```python
from build123d import *

# Parameters (mm, degrees)
CROQUIS1_R              = 17.985951022
SALIENTE_EXTRUIR1_DEPTH = 3


with BuildPart() as part:
    # Croquis1 → Saliente-Extruir1 (new body)
    with BuildSketch(Plane.XY):
        with BuildLine():
            Line((69.938444675, 17.671179984), (59.198401062, 17.671179984))
            Line((59.198401062, 17.671179984), (59.198401062, 32.584255723))
            ThreePointArc((59.198401062, 32.584255723), (65.364018559, 84.900042365), (69.938444675, 32.421179984))
            Line((69.938444675, 32.421179984), (69.938444675, 26.421179984))
            Line((69.938444675, 26.421179984), (64.938444675, 26.421179984))
            Line((64.938444675, 26.421179984), (64.938444675, 23.671179984))
            Line((64.938444675, 23.671179984), (69.938444675, 23.671179984))
            Line((69.938444675, 23.671179984), (69.938444675, 17.671179984))
        make_face()
        with Locations((64.962042446, 58.426202565)):
            Circle(CROQUIS1_R, mode=Mode.SUBTRACT)
    extrude(amount=SALIENTE_EXTRUIR1_DEPTH)


solid = part.part
```
The model under review builds one solid part; all positions refer to its coordinate system, in mm. A direction names the side the tool comes from. Round coordinates to 2 decimals unless told otherwise and drop trailing zeros. Order: outer loops, then holes, each group sorted by start corner. A loop starts at its lowest first (then second) coordinate and runs counter-clockwise, first axis right, second up. Notation, with made-up numbers: (-9, 59) -> (46, 59) arc R12 ccw to (46, 70) -> close; hole circle Ø5 at (37.5, -2.5). An arc over 180 degrees is marked (long way). One line per item, written item: value. Start each with the question number.
Q1. Take a section at A-A (x = 54.5). Write out the cut boundary in (y, z).
Q2. Wall thickness on line 1 (Y direction, x = 57.5, z = 1); line 2 (Y direction, x = 50, z = 0.6); line 3 (X direction, y = 59, z = 1.5): over which ranges is each line inside the solid? List them lowest first.
Q3. Mouldability with a two-part tool opening along Y and no side actions: class faces 1 (the face through (64.938, 25, 1)), 2 (the face through (59.198, 25, 1)), 3 (the face through (65, 17.671, 1)) as released by +Y, released by -Y, zero draft, split by the parting line, or undercut.
Q4. Take a section at B-B (y = 50). Write out the cut boundary in (x, z), and give its area (3 significant figures).
Q5. Take a section at C-C (z = 0.6). Write out the cut boundary in (x, y).
Q6. Take a section at D-D (x = 44). Write out the cut boundary in (y, z), and give its area (3 significant figures).
Q7. Clearance check with flat-ended pins moving along their axes: pin 1 Ø1 at (y, z) = (42.5, 0.5) entering from -X; pin 2 Ø0.9 at (y, z) = (22, 1.5) entering from +X; pin 3 Ø1 at (y, z) = (62, 1.5) entering from -X. State where each tip first meets the part, or that it passes through.
Q8. Machinability: for faces 4 (the face through (69.938, 21, 1)), 5 (the face through (67, 23.671, 1)), 6 (the face through (77, 44, 0)), which of the approach directions +Z, -Z, +X, -X, +Y, -Y give a long, thin tool a straight path to every point of the face, cutting with its end or side? Answer none if there is none.
Reported:
1. outline: (34.1, 0) -> (43.8, 0) -> (43.8, 3) -> (34.1, 3) -> close; (73.06, 0) -> (82.75, 0) -> (82.75, 3) -> (73.06, 3) -> close
2. line 1: y = 33.02 to 42.06, 74.79 to 83.83
2. line 2: y = 36.58 to 48.44, 68.41 to 80.27
2. line 3: x = 38.49 to 46.99, 82.94 to 91.43
3. face 1: undercut
3. face 2: zero draft
3. face 3: released by -Y
4. outline: (39.86, 0) -> (49.07, 0) -> (49.07, 3) -> (39.86, 3) -> close; (80.85, 0) -> (90.06, 0) -> (90.06, 3) -> (80.85, 3) -> close
4. area: 55.3 mm2
5. outline: (59.2, 17.67) -> (69.94, 17.67) -> (69.94, 23.67) -> (64.94, 23.67) -> (64.94, 26.42) -> (69.94, 26.42) -> (69.94, 32.42) arc R26.48 ccw (long way) to (59.2, 32.58) -> close; hole circle Ø35.97 at (64.96, 58.43)
6. outline: (42.25, 0) -> (74.6, 0) -> (74.6, 3) -> (42.25, 3) -> close
6. area: 97.0 mm2
7. pin 1: stops at x = 43.44
7. pin 2: stops at x = 69.94
7. pin 3: stops at x = 38.66
8. face 4: +Z, -Z, +X, -Y
8. face 5: +Z, -Z, +X
8. face 6: -Z, +X, -X, +Y, -Y
